The listing builds one solid part. Answer for the finished solid, in the listing's coordinates (mm). Face numbers are marked on the shaded views. A direction names the side the tool comes from. Coordinates: 2 decimals unless noted, no trailing zeros. Order: outer loops, then holes, each group sorted by start corner. A loop starts at its lowest first (then second) coordinate and runs counter-clockwise, first axis right, second up. Notation, with made-up numbers: (34, 43.5) - (75, 43.5) arc R25 ccw to (75, 82.5) - close; hole circle Ø3 at (45.25, 34.25). An arc over 180 degrees is marked (long way). Use a Markdown table: item, result. Add a question column.
Item 1: For the marked faces 1 and 2, determine the directions among +Z, -Z, +X, -X, +Y, -Y from which every point of the face is accessible in a straight line to the end or side of a thin tool.
Item 2: The part is cut by section A-A, the plane z = 2.75. Give the vertices of the cut face in (x, y), then the cut area to 3 significant figures.
Item 3: The part is cut by section C-C, the plane z = -3. Give the vertices of the cut face in (x, y).
Item 4: Find the intervals of material crossed by line 1 along X through (y, z) = (-0.2, 3.25); line 2 along X through (y, z) = (-0.85, 0.5); line 3 along Z through (x, y) = (0.25, 0.9), in increasing order.
Item 5: The mould has two halves that part along X. Classify the marked faces 3, 4 and 5: released by +X, released by -X, zero draft, split by the parting line, or undercut.
Item 6: Flat-ended cylindrical pins translate along their axes: P1, Ø2, axis at x = 0, y = 0, coming from the +Z side; P2, Ø2, axis at y = -1.5, z = -1.5, coming from the -X side. Find the tip coordinate at first contact, or state that the pin passes through.
Item 7: The part is cut by section B-B, the plane x = 0. Give the vertices of the cut face in (y, z) (3 decimals).
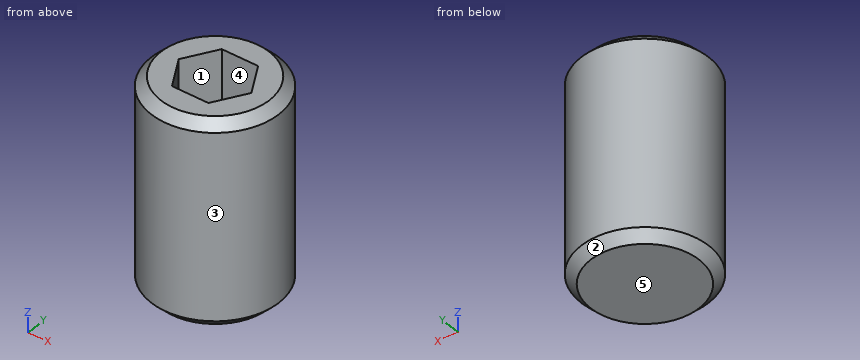
Solid Edge part; units mm, degrees
sketch "Sketch1" plane through (0, 0, 0) normal (0, 0, 1) x (1, 0, 0)
  circle A0 centre (0, 0) radius 2.5
extrude "Protrusion1" add sketch "Sketch1" along normal mid plane 8
chamfer "Chamfer1" distance 0.375 angle 45 2 edges at (-2.5, 0, -4) (-2.5, 0, 4)
sketch "Sketch2" plane through (0, 0, 4) normal (0, 0, 1) x (1, 0, 0)
  line L0 (-0.7217, 1.25) -> (0.7217, 1.25)
  line L1 (1.4434, 0) -> (0.7217, 1.25)
  line L2 (0.7217, -1.25) -> (1.4434, 0)
  line L3 (-0.7217, -1.25) -> (0.7217, -1.25)
  line L4 (-1.4434, 0) -> (-0.7217, -1.25)
  line L5 (-0.7217, 1.25) -> (-1.4434, 0)
extrude "Cutout1" cut sketch "Sketch2" against normal blind 4
properties part number "24105901"
Solution:
| question | item | result |
|---|---|---|
| 1 | face 1 | +Z |
| 1 | face 2 | -Z |
| 2 | outline | circle Ø5 at (0, 0); hole (-1.44, 0) - (-0.72, -1.25) - (0.72, -1.25) - (1.44, 0) - (0.72, 1.25) - (-0.72, 1.25) - close |
| 2 | area | 14.2 mm2 |
| 3 | outline | circle Ø5 at (0, 0) |
| 4 | line 1 | x = -2.49 to -1.33, 1.33 to 2.49 |
| 4 | line 2 | x = -2.35 to -0.95, 0.95 to 2.35 |
| 4 | line 3 | z = -4 to 0 |
| 5 | face 3 | split by the parting line |
| 5 | face 4 | undercut |
| 5 | face 5 | zero draft |
| 6 | P1 | stops at z = 0 |
| 6 | P2 | stops at x = -2.45 |
| 7 | outline | (-2.5, -3.625) - (-2.125, -4) - (2.125, -4) - (2.5, -3.625) - (2.5, 3.625) - (2.125, 4) - (1.25, 4) - (1.25, 0) - (-1.25, 0) - (-1.25, 4) - (-2.125, 4) - (-2.5, 3.625) - close |
